Source: three-view drawing plus pictorial views. Frame: mm from the lowest corner of the part. A direction names the side the tool comes from. Give positions to 0.01 mm unless a question says otherwise; leave off trailing zeros. Loops run counter-clockwise (first coordinate to the right, second up) from the corner with the lowest first, then second, coordinate; pieces in that order, holes last.
1. Section C-C, the plane z = 32.5. Output: boundary loops of the cut face in (x, y), then the cut area to 3 significant figures.
2. Section B-B, the plane y = 14. Output: boundary loops of the cut face in (x, z).
3. First-contact query: P1, Ø1, axis at x = 37.5, z = 24, coming from the +Y side; P2, Ø5, axis at x = 26, z = 5, coming from the +Y side; P3, Ø4, axis at y = 56, z = 33.5, coming from the -X side. Flat tips, straight axial feed; report the tip coordinate or a pass-through.
4. Draft query along Z for the marked faces 1, 2, 3 and 4. Return one class per face: +Z half, -Z half, draft (parallel to the pull), parting line (faces both ways), or undercut.
5. Access query for the marked faces 5, 6 and 7. Directions: +Z, -Z, +X, -X, +Y, -Y. A direction counts if a zero-diameter tool reaches every point of the face in a straight line with its end or side. Return the directions, or none.
6. Section A-A, the plane x = 25. Output: boundary loops of the cut face in (y, z).
7. Section D-D, the plane y = 28. Output: boundary loops of the cut face in (x, z).
8. Material intervals for line 1 along Z through (x, y) = (23, 21); line 2 along Y through (x, z) = (25, 4); line 3 along Z through (x, y) = (26.5, 36), sorted ascending.
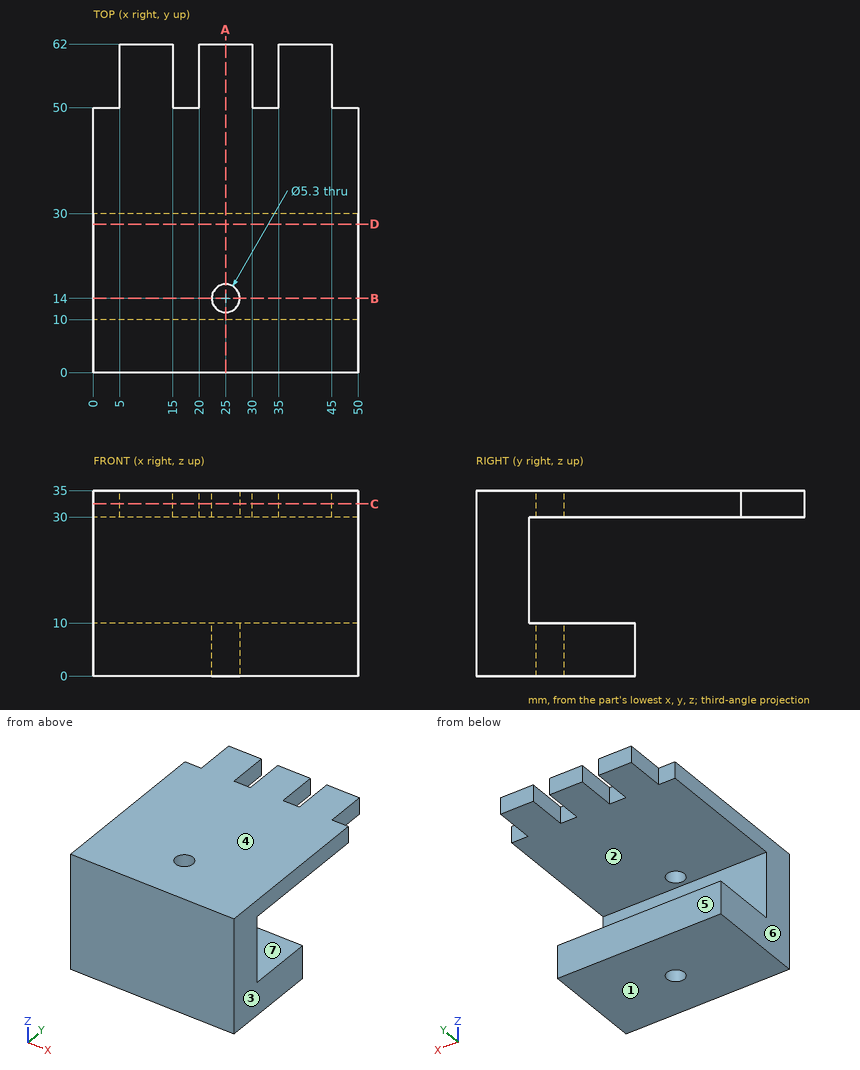
Answers below:
1. outline: (0, 0) - (50, 0) - (50, 50) - (45, 50) - (45, 62) - (35, 62) - (35, 50) - (30, 50) - (30, 62) - (20, 62) - (20, 50) - (15, 50) - (15, 62) - (5, 62) - (5, 50) - (0, 50) - close; hole circle Ø5.3 at (25, 14)
1. area: 2,840 mm2
2. outline: (0, 0) - (22.35, 0) - (22.35, 10) - (0, 10) - close; (0, 30) - (22.35, 30) - (22.35, 35) - (0, 35) - close; (27.65, 0) - (50, 0) - (50, 10) - (27.65, 10) - close; (27.65, 30) - (50, 30) - (50, 35) - (27.65, 35) - close
3. P1: stops at y = 10
3. P2: stops at y = 30
3. P3: stops at x = 5
4. face 1: -Z half
4. face 2: undercut
4. face 3: draft
4. face 4: +Z half
5. face 5: -Z, +X, -X, +Y
5. face 6: +Z, -Z, -X, +Y, -Y
5. face 7: +X, -X, +Y
6. outline: (0, 0) - (11.35, 0) - (11.35, 10) - (10, 10) - (10, 30) - (11.35, 30) - (11.35, 35) - (0, 35) - close; (16.65, 0) - (30, 0) - (30, 10) - (16.65, 10) - close; (16.65, 30) - (62, 30) - (62, 35) - (16.65, 35) - close
7. outline: (0, 0) - (50, 0) - (50, 10) - (0, 10) - close; (0, 30) - (50, 30) - (50, 35) - (0, 35) - close
8. line 1: z = 0 to 10, 30 to 35
8. line 2: y = 0 to 11.35, 16.65 to 30
8. line 3: z = 30 to 35
